Geometry check sheet. Reference: the model listing, model coordinates, mm. Round coordinates to 2 decimals unless told otherwise and drop trailing zeros. Write each loop counter-clockwise with the first axis right and the second up, starting at its lowest first coordinate (ties: lowest second). Pieces come first, ordered by that corner, then holes. Notation, with made-up numbers: M 23.25,46 L 67.25,46 A30 cw 67.25,82 Z; hole C 45.25,-7 d3. An arc over 180 degrees is marked long. One line per item, written item: value. Start each with the question number.
1. Scan lines: probe 1 along Z at (x, y) = (-5.5, -9.5); probe 2 along X at (y, z) = (-5, -12.25); probe 3 along Y at (x, z) = (-2, -12.75). Record each from-to range of solid material in increasing order. Write a range as [from, to].
2. Release check for a two-part mould opening along X. For faces 1 (the flat face through (-4.7, -5.8, -20.77)), 2 (the flat face through (-7.2, -0.2, -16.696)) record: pulls with the +X half, pulls with the -X half, needs draft (parallel to the pull), parting line crosses it, or undercut.
3. Section check A-A (z = -14.75). Record the boundary of the cut face in (x, y), and give its area (3 significant figures).
4. Depth check by flat-ended pin: P1, Ø1, axis at x = -7, y = 2.5, coming from the -Z side; P2, Ø1.3, axis at x = -5.5, y = -6, coming from the -Z side; P3, Ø5, axis at y = -3.5, z = -17.5, coming from the -X side. Enter the tip coordinate at first touch or a pass-through.
from build123d import *

# Parameters (mm, degrees)
REDONDEO3_R           = 0.7
REDONDEO5_R           = 1.5
CROQUIS2_R            = 2.5
CROQUIS2_R_2          = 1.5
CORTAR_EXTRUIR1_DEPTH = 3
CORTAR_EXTRUIR3_DEPTH = 3


# Read off the part's stored shape, not the designer's step: Sólido-Eliminar/Conservar 1
with BuildPart() as part:
    # Croquis1 → Revolución1 (revolve)
    with BuildSketch(Plane(origin=(0, 0, 0), x_dir=(0, 0, -1), z_dir=(1, 0, 0)), mode=Mode.PRIVATE) as revoluci_n1_sk:
        with BuildLine():
            Line((10.5, 4), (12.997954185, 4))
            Line((12.997954185, 4), (13.5, 3.497954185))
            Line((13.5, 3.497954185), (13.5, 0))
            Line((13.5, 0), (25.5, 0))
            ThreePointArc((25.5, 0), (25.166294504, 2.428032035), (24.189924541, 4.676009041))
            Line((24.189924541, 4.676009041), (16.696080767, 17))
            Line((16.696080767, 17), (16.696080767, 7))
            Line((16.696080767, 7), (10.5, 7))
            Line((10.5, 7), (10.5, 4))
        make_face()
    revolve(revoluci_n1_sk.sketch.rotate(Axis((0, 0, 43.421280629), (0, 0, -1)), 90), axis=Axis((0, 0, 43.421280629), (0, 0, -1)))

    # Redondeo3
    redondeo3_edges = [part.edges().sort_by_distance(p)[0] for p in [
        (-4, 0, -10.5),
    ]]
    fillet(redondeo3_edges, radius=REDONDEO3_R)

    # Redondeo5
    redondeo5_edges = [part.edges().sort_by_distance(p)[0] for p in [
        (-17, 0, -16.696080767),
        (-7, 0, -10.5),
    ]]
    fillet(redondeo5_edges, radius=REDONDEO5_R)

    # Croquis2 → Cortar-Extruir1 (cut)
    # profile 1 of 5: a face of its own
    with BuildSketch(Plane(origin=(0, 0, -25.5), x_dir=(-1, 0, 0), z_dir=(0, 0, -1))):
        Circle(CROQUIS2_R)
        Circle(CROQUIS2_R_2, mode=Mode.SUBTRACT)
    # profile 2 of 5: a face of its own
    with BuildSketch(Plane(origin=(0, 0, -25.5), x_dir=(-1, 0, 0), z_dir=(0, 0, -1))):
        with BuildLine():
            Line((-0.35, 2.677218706), (0.557333453, 4.114836877))
            Line((0.557333453, 4.114836877), (-0.216020438, 3.677218706))
            Line((-0.216020438, 3.677218706), (1.01365522, 5.207218706))
            Line((1.01365522, 5.207218706), (0.420313019, 4.267101787))
            Line((0.420313019, 4.267101787), (0.85, 4.510248984))
            Line((0.85, 4.510248984), (0.35, 2.677218706))
            ThreePointArc((0.35, 2.677218706), (0, 2.7), (-0.35, 2.677218706))
        make_face()
    # profile 3 of 5: a face of its own
    with BuildSketch(Plane(origin=(0, 0, -25.5), x_dir=(-1, 0, 0), z_dir=(0, 0, -1))):
        with BuildLine():
            Line((4.510248984, -0.85), (2.677218706, -0.35))
            ThreePointArc((2.677218706, -0.35), (2.7, 0), (2.677218706, 0.35))
            Line((2.677218706, 0.35), (4.114836877, -0.557333453))
            Line((4.114836877, -0.557333453), (3.677218706, 0.216020438))
            Line((3.677218706, 0.216020438), (5.207218706, -1.01365522))
            Line((5.207218706, -1.01365522), (4.267101787, -0.420313019))
            Line((4.267101787, -0.420313019), (4.510248984, -0.85))
        make_face()
    # profile 4 of 5: a face of its own
    with BuildSketch(Plane(origin=(0, 0, -25.5), x_dir=(-1, 0, 0), z_dir=(0, 0, -1))):
        with BuildLine():
            Line((-0.85, -4.510248984), (-0.35, -2.677218706))
            ThreePointArc((-0.35, -2.677218706), (0, -2.7), (0.35, -2.677218706))
            Line((0.35, -2.677218706), (-0.557333453, -4.114836877))
            Line((-0.557333453, -4.114836877), (0.216020438, -3.677218706))
            Line((0.216020438, -3.677218706), (-1.01365522, -5.207218706))
            Line((-1.01365522, -5.207218706), (-0.420313019, -4.267101787))
            Line((-0.420313019, -4.267101787), (-0.85, -4.510248984))
        make_face()
    # profile 5 of 5: a face of its own
    with BuildSketch(Plane(origin=(0, 0, -25.5), x_dir=(-1, 0, 0), z_dir=(0, 0, -1))):
        with BuildLine():
            Line((-4.510248984, 0.85), (-2.677218706, 0.35))
            ThreePointArc((-2.677218706, 0.35), (-2.7, 0), (-2.677218706, -0.35))
            Line((-2.677218706, -0.35), (-4.114836877, 0.557333453))
            Line((-4.114836877, 0.557333453), (-3.677218706, -0.216020438))
            Line((-3.677218706, -0.216020438), (-5.207218706, 1.01365522))
            Line((-5.207218706, 1.01365522), (-4.267101787, 0.420313019))
            Line((-4.267101787, 0.420313019), (-4.510248984, 0.85))
        make_face()
    extrude(amount=-CORTAR_EXTRUIR1_DEPTH, mode=Mode.SUBTRACT)

    # Croquis3 → Cortar-Extruir3 (cut)
    with BuildSketch(Plane.XY.offset(-23.77)):
        with BuildLine():
            Line((-0.35, 6.666828085), (0.557333453, 8.104446256))
            Line((0.557333453, 8.104446256), (-0.216020438, 7.666828085))
            Line((-0.216020438, 7.666828085), (1.01365522, 9.196828085))
            Line((1.01365522, 9.196828085), (0.420313019, 8.256711166))
            Line((0.420313019, 8.256711166), (0.85, 8.499858363))
            Line((0.85, 8.499858363), (0.35, 6.666828085))
            ThreePointArc((0.35, 6.666828085), (0, 6.676009041), (-0.35, 6.666828085))
        make_face()
        with BuildLine():
            Line((3.63550728, 5.599302058), (5.214566222, 6.229042367))
            Line((5.214566222, 6.229042367), (4.331684274, 6.329567842))
            Line((4.331684274, 6.329567842), (6.225824216, 6.844578626))
            Line((6.225824216, 6.844578626), (5.193213431, 6.432765857))
            Line((5.193213431, 6.432765857), (5.683755838, 6.376912401))
            Line((5.683755838, 6.376912401), (4.201819176, 5.187852381))
            ThreePointArc((4.201819176, 5.187852381), (3.924059658, 5.401004769), (3.63550728, 5.599302058))
        make_face()
        with BuildLine():
            Line((6.232374345, 2.393032958), (7.880011931, 1.974356011))
            Line((7.880011931, 1.974356011), (7.224832823, 2.574627817))
            Line((7.224832823, 2.574627817), (9.059939969, 1.87793277))
            Line((9.059939969, 1.87793277), (7.982482824, 2.151722632))
            Line((7.982482824, 2.151722632), (8.346510129, 1.818202645))
            Line((8.346510129, 1.818202645), (6.448686241, 1.727293396))
            ThreePointArc((6.448686241, 1.727293396), (6.349261901, 2.063000248), (6.232374345, 2.393032958))
        make_face()
        with BuildLine():
            Line((6.448686241, -1.727293396), (7.535560914, -3.034467235))
            Line((7.535560914, -3.034467235), (7.358340796, -2.163732526))
            Line((7.358340796, -2.163732526), (8.43346659, -3.806019575))
            Line((8.43346659, -3.806019575), (7.722715092, -2.951205504))
            Line((7.722715092, -2.951205504), (7.821181238, -3.434998723))
            Line((7.821181238, -3.434998723), (6.232374345, -2.393032958))
            ThreePointArc((6.232374345, -2.393032958), (6.349261901, -2.063000248), (6.448686241, -1.727293396))
        make_face()
        with BuildLine():
            Line((4.201819176, -5.187852381), (4.312781752, -6.884227135))
            Line((4.312781752, -6.884227135), (4.681212686, -6.075620586))
            Line((4.681212686, -6.075620586), (4.585695617, -8.036201804))
            Line((4.585695617, -8.036201804), (4.513132681, -6.926873445))
            Line((4.513132681, -6.926873445), (4.308426947, -7.37614733))
            Line((4.308426947, -7.37614733), (3.63550728, -5.599302058))
            ThreePointArc((3.63550728, -5.599302058), (3.924059658, -5.401004769), (4.201819176, -5.187852381))
        make_face()
        with BuildLine():
            Line((0.35, -6.666828085), (-0.557333453, -8.104446256))
            Line((-0.557333453, -8.104446256), (0.216020438, -7.666828085))
            Line((0.216020438, -7.666828085), (-1.01365522, -9.196828085))
            Line((-1.01365522, -9.196828085), (-0.420313019, -8.256711166))
            Line((-0.420313019, -8.256711166), (-0.85, -8.499858363))
            Line((-0.85, -8.499858363), (-0.35, -6.666828085))
            ThreePointArc((-0.35, -6.666828085), (0, -6.676009041), (0.35, -6.666828085))
        make_face()
        with BuildLine():
            Line((-3.63550728, -5.599302058), (-5.214566222, -6.229042367))
            Line((-5.214566222, -6.229042367), (-4.331684274, -6.329567842))
            Line((-4.331684274, -6.329567842), (-6.225824216, -6.844578626))
            Line((-6.225824216, -6.844578626), (-5.193213431, -6.432765857))
            Line((-5.193213431, -6.432765857), (-5.683755838, -6.376912401))
            Line((-5.683755838, -6.376912401), (-4.201819176, -5.187852381))
            ThreePointArc((-4.201819176, -5.187852381), (-3.924059658, -5.401004769), (-3.63550728, -5.599302058))
        make_face()
        with BuildLine():
            Line((-6.232374345, -2.393032958), (-7.880011931, -1.974356011))
            Line((-7.880011931, -1.974356011), (-7.224832823, -2.574627817))
            Line((-7.224832823, -2.574627817), (-9.059939969, -1.87793277))
            Line((-9.059939969, -1.87793277), (-7.982482824, -2.151722632))
            Line((-7.982482824, -2.151722632), (-8.346510129, -1.818202645))
            Line((-8.346510129, -1.818202645), (-6.448686241, -1.727293396))
            ThreePointArc((-6.448686241, -1.727293396), (-6.349261901, -2.063000248), (-6.232374345, -2.393032958))
        make_face()
        with BuildLine():
            Line((-6.448686241, 1.727293396), (-7.535560914, 3.034467235))
            Line((-7.535560914, 3.034467235), (-7.358340796, 2.163732526))
            Line((-7.358340796, 2.163732526), (-8.43346659, 3.806019575))
            Line((-8.43346659, 3.806019575), (-7.722715092, 2.951205504))
            Line((-7.722715092, 2.951205504), (-7.821181238, 3.434998723))
            Line((-7.821181238, 3.434998723), (-6.232374345, 2.393032958))
            ThreePointArc((-6.232374345, 2.393032958), (-6.349261901, 2.063000248), (-6.448686241, 1.727293396))
        make_face()
        with BuildLine():
            Line((-4.201819176, 5.187852381), (-4.312781752, 6.884227135))
            Line((-4.312781752, 6.884227135), (-4.681212686, 6.075620586))
            Line((-4.681212686, 6.075620586), (-4.585695617, 8.036201804))
            Line((-4.585695617, 8.036201804), (-4.513132681, 6.926873445))
            Line((-4.513132681, 6.926873445), (-4.308426947, 7.37614733))
            Line((-4.308426947, 7.37614733), (-3.63550728, 5.599302058))
            ThreePointArc((-3.63550728, 5.599302058), (-3.924059658, 5.401004769), (-4.201819176, 5.187852381))
        make_face()
    extrude(amount=CORTAR_EXTRUIR3_DEPTH, mode=Mode.SUBTRACT)


with BuildPart() as body_2:
    # Partir1: the piece on the far side of the plane
    add(part.part)
    split(bisect_by=Plane(origin=(0, 0, 0), x_dir=(0, 0, 1), z_dir=(1, 0, 0)), keep=Keep.BOTTOM)


with BuildPart() as part_1:
    add(part.part)

    # Partir1
    split(bisect_by=Plane(origin=(0, 0, 0), x_dir=(0, 0, 1), z_dir=(1, 0, 0)), keep=Keep.TOP)


solid = body_2.part
Result sheet:
1. probe 1: z = [-20.36, -16.7]
1. probe 2: x = [-4.9, 0]
1. probe 3: y = [-6.71, -3.46], [3.46, 6.71]
2. face 1: undercut
2. face 2: needs draft
3. outline: M 0,-7 L 0,7 A7 ccw Z
3. area: 77.0 mm2
4. P1: stops at z = -22.78
4. P2: stops at z = -22.48
4. P3: stops at x = -13.1
